Can you work these out from the model? Positions are in its coordinate system, mm. A direction names the side the tool comes from. Coordinates: 2 decimals unless noted, no trailing zeros. Loops run counter-clockwise (first coordinate to the right, second up) from the corner with the lowest first, then second, coordinate; pieces in that order, holes last. Notation, with made-up numbers: M 51,-13 L 80,-13 A24 ccw 80,21 Z; hole C 73,47 d9. An arc over 180 degrees is marked long. Answer as a JSON object with one key per item and string values. Group by question number.
Item 1: Suppose I cut it at C-C (x = -31.5). Write out the boundary of the cut face in (y, z), then the cut area to 3 significant figures.
Item 2: I'm going to push flat-ended pins straight in: pin 1 Ø5 at (x, z) = (-26.5, 28.5) entering from -Y; pin 2 Ø0.9 at (y, z) = (1, 5) entering from +X; pin 3 Ø1.5 at (x, y) = (-22.5, 1.5) entering from +Z; pin 4 Ø1.5 at (y, z) = (2, 22.5) entering from -X. Where does each tip first touch, or does it pass through?
Item 3: Suppose I cut it at B-B (z = 32.5). Write out the boundary of the cut face in (x, y).
Item 4: Suppose I cut it at A-A (x = -7.5). Write out the boundary of the cut face in (y, z).
Item 5: Suppose I cut it at D-D (y = 0.9). Write out the boundary of the cut face in (x, z).
Item 6: If I drill on line 1 (X direction, y = 1.95, z = 7.5); line 2 (X direction, y = 1.6, z = 22.5); line 3 (X direction, y = 0.95, z = 12.5), over which ranges is the centre line in solid material (lowest first)?
Item 7: Which directions (+Z, -Z, +X, -X, +Y, -Y) give clear straight access to the entire face, cutting with the end or side of a thin tool? Please do faces 1 (the cylindrical face through (-26.02, 1.48, 16.2)), 2 (the flat face through (-15, 1, 22)), 3 (the cylindrical face through (-17.57, 1.48, 14.4)), 4 (the flat face through (-17, 2, 8)).
Item 8: We'd pull the mould along Z, two halves only. Please class faces 5 (the flat face through (-26.4, 1.5, 26.1)), 6 (the cylindrical face through (-16.27, 1.48, 26.05)), 7 (the flat face through (-19, 0, 14)), 8 (the cylindrical face through (-36.93, 1.52, 0.6)): +Z half, -Z half, draft (parallel to the pull), parting line (faces both ways), or undercut.
```python
from build123d import *

# Parameters (mm, degrees)
SKETCH_1_R          = 1.45
EXTRUDE_1_DEPTH     = 3
EXTRUDE_2_DEPTH     = 3
SKETCH_3_W          = 17
SKETCH_3_H          = 17
CUT_EXTRUDE_1_DEPTH = 54.117793629
FILLET_1_R          = 2


with BuildPart() as part:
    # 草图1 → 凸台-拉伸1 (new body)
    with BuildSketch(Plane(origin=(0, 0, 0), x_dir=(1, 0, 0), z_dir=(0, 1, 0))):
        Polygon((0, 0), (-37.5, 0), (-37.5, -15), (-15, -15), (-15, -37.5), (0, -37.5), align=None)
        with Locations(Location((-7.5, -7.5, 0), (0, 0, 270))):
            Circle(SKETCH_1_R, mode=Mode.SUBTRACT)
        with Locations(Location((-22.5, -7.5, 0), (0, 0, 270))):
            Circle(SKETCH_1_R, mode=Mode.SUBTRACT)
        with Locations(Location((-32.5, -7.5, 0), (0, 0, 270))):
            Circle(SKETCH_1_R, mode=Mode.SUBTRACT)
        with Locations(Location((-7.5, -22.5, 0), (0, 0, 270))):
            Circle(SKETCH_1_R, mode=Mode.SUBTRACT)
        with Locations(Location((-7.5, -32.5, 0), (0, 0, 270))):
            Circle(SKETCH_1_R, mode=Mode.SUBTRACT)
    extrude(amount=EXTRUDE_1_DEPTH)

    # 草图2 → 凸台-拉伸2 (add)
    with BuildSketch(Plane(origin=(0, 3, 0), x_dir=(1, 0, 0), z_dir=(0, 1, 0))):
        Polygon((-37.5, -15), (-15, -37.5), (-15, -29.014718626), (-29.014718626, -15), align=None)
    extrude(amount=-EXTRUDE_2_DEPTH)

    # 草图3 → 切除-拉伸1 (cut, through all)
    with BuildSketch(Plane(origin=(0, 3, 0), x_dir=(1, 0, 0), z_dir=(0, 1, 0))):
        with Locations((-8.5, -8.5)):
            Rectangle(SKETCH_3_W, SKETCH_3_H)
    extrude(amount=-CUT_EXTRUDE_1_DEPTH, mode=Mode.SUBTRACT)

    # 圆角1
    fillet_1_edges = [part.edges().sort_by_distance(p)[0] for p in [
        (0, 1.5, 37.5),
        (-15, 1.5, 37.5),
        (-37.5, 1.5, 15),
        (-37.5, 1.5, 0),
        (-29.014718626, 1.5, 15),
        (-15, 1.5, 29.014718626),
        (-15, 1.5, 17),
        (-17, 1.5, 15),
        (0, 1.5, 17),
        (-17, 1.5, 0),
    ]]
    fillet(fillet_1_edges, radius=FILLET_1_R)


solid = part.part
```
From the geometry:
{
 "1": {"outline": "M 0,0 L 3,0 L 3,6.45 L 0,6.45 Z; M 0,8.55 L 3,8.55 L 3,21 L 0,21 Z", "area": "56.7 mm2"},
 "2": {"pin 1": "y = 0", "pin 2": "x = -17", "pin 3": "z = 30.75", "pin 4": "x = -30.75"},
 "3": {"outline": "M -20,0 L -8.95,0 L -8.95,3 L -20,3 Z; M -6.05,0 L 0,0 L 0,3 L -6.05,3 Z"},
 "4": {"outline": "M 0,17 L 3,17 L 3,21.05 L 0,21.05 Z; M 0,23.95 L 3,23.95 L 3,31.05 L 0,31.05 Z; M 0,33.95 L 3,33.95 L 3,37.5 L 0,37.5 Z"},
 "5": {"outline": "M -37.5,2 A2 ccw -35.5,0 L -19,0 A2 ccw -17,2 L -17,13 A2 ccw -19,15 L -24.19,15 A2 cw -25.6,18.41 L -18.41,25.6 A2 cw -15,24.19 L -15,19 A2 ccw -13,17 L -2,17 A2 ccw 0,19 L 0,35.5 A2 ccw -2,37.5 L -14.17,37.5 A2 ccw -15.59,36.91 L -36.91,15.59 A2 ccw -37.5,14.17 Z; hole C -32.5,7.5 d2.9; hole C -22.5,7.5 d2.9; hole C -7.5,22.5 d2.9; hole C -7.5,32.5 d2.9"},
 "6": {"line 1": "-37.5 to -33.95, -31.05 to -23.95, -21.05 to -17", "line 2": "-30 to -21.51, -15 to -8.95, -6.05 to 0", "line 3": "-37.5 to -17"},
 "7": {"face 1": "+Y, -Y", "face 2": "-Z, +Y, -Y", "face 3": "+X, +Y, -Y", "face 4": "-Z, +X, +Y, -Y"},
 "8": {"face 5": "+Z half", "face 6": "undercut", "face 7": "draft", "face 8": "-Z half"}
}
